Geometry check sheet. Reference: the model listing, model coordinates, mm. Give positions to 0.01 mm unless a question says otherwise; leave off trailing zeros. Write each loop counter-clockwise with the first axis right and the second up, starting at its lowest first coordinate (ties: lowest second). Pieces come first, ordered by that corner, then holes. Notation, with made-up numbers: (-39, 80.25) - (2, 80.25) arc R17 ccw to (2, 99.25) - close; hole circle Ø10 at (24.25, 77.5). An arc over 180 degrees is marked (long way). Use a Markdown table: item, result.
```python
from build123d import *

# Parameters (mm, degrees)
SKETCH1_W           = 82.55
SKETCH1_H           = 83.82
BOSS_EXTRUDE1_DEPTH = 19.05
SKETCH2_R           = 0.889
CUT_EXTRUDE1_DEPTH  = 71.083405489
FILLET1_R           = 2.54
SKETCH3_R           = 3.175
CUT_EXTRUDE2_DEPTH  = 38.1


with BuildPart() as part:
    # Sketch1 → Boss-Extrude1 (new, symmetric)
    with BuildSketch(Plane.XY):
        Rectangle(SKETCH1_W, SKETCH1_H)
    extrude(amount=BOSS_EXTRUDE1_DEPTH, both=True)

    # Sketch2 → Cut-Extrude1 (cut, through all)
    with BuildSketch(Plane.XY.offset(19.05)):
        with Locations((-28.575, 29.845)):
            Circle(SKETCH2_R)
        with Locations((28.575, 29.845)):
            Circle(SKETCH2_R)
        with Locations((28.575, 1.27)):
            Circle(SKETCH2_R)
        with Locations((-28.575, 1.27)):
            Circle(SKETCH2_R)
        with Locations((-19.685, 1.27)):
            Circle(SKETCH2_R)
        with Locations((19.685, 1.27)):
            Circle(SKETCH2_R)
    extrude(amount=-CUT_EXTRUDE1_DEPTH, mode=Mode.SUBTRACT)

    # Fillet1
    fillet1_edges = [part.edges().sort_by_distance(p)[0] for p in [
        (-41.275, 0, 19.05),
        (41.275, 0, 19.05),
        (-41.275, 0, -19.05),
        (41.275, 0, -19.05),
    ]]
    fillet(fillet1_edges, radius=FILLET1_R)

    # Sketch3 → Cut-Extrude2 (cut)
    with BuildSketch(Plane(origin=(0, 41.91, 0), x_dir=(1, 0, 0), z_dir=(0, 1, 0))):
        with Locations(Location((-6.35, 0, 0), (0, 0, 270))):
            Circle(SKETCH3_R)
        with Locations(Location((6.35, 0, 0), (0, 0, 270))):
            Circle(SKETCH3_R)
        with Locations(Location((19.05, 0, 0), (0, 0, 270))):
            Circle(SKETCH3_R)
        with Locations(Location((-19.05, 0, 0), (0, 0, 270))):
            Circle(SKETCH3_R)
    extrude(amount=-CUT_EXTRUDE2_DEPTH, mode=Mode.SUBTRACT)


solid = part.part
```
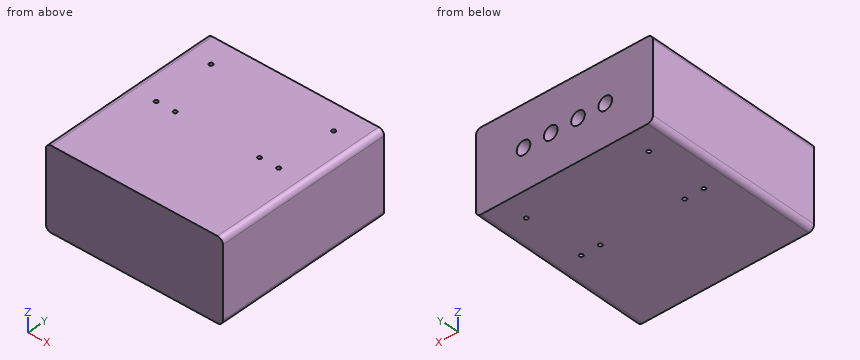
1) Section check C-C on x = -6.35. Record the boundary of the cut face in (y, z) (3 decimals).
Working result:
| item | result |
|---|---|
| outline | (-41.91, -19.05) - (41.91, -19.05) - (41.91, -3.175) - (3.81, -3.175) - (3.81, 3.175) - (41.91, 3.175) - (41.91, 19.05) - (-41.91, 19.05) - close |
2) Section check B-B on z = 0. Record the boundary of the cut face in (x, y) (3 decimals).
Working result:
| item | result |
|---|---|
| outline | (-41.275, -41.91) - (41.275, -41.91) - (41.275, 41.91) - (22.225, 41.91) - (22.225, 3.81) - (15.875, 3.81) - (15.875, 41.91) - (9.525, 41.91) - (9.525, 3.81) - (3.175, 3.81) - (3.175, 41.91) - (-3.175, 41.91) - (-3.175, 3.81) - (-9.525, 3.81) - (-9.525, 41.91) - (-15.875, 41.91) - (-15.875, 3.81) - (-22.225, 3.81) - (-22.225, 41.91) - (-41.275, 41.91) - close; hole circle Ø1.778 at (-28.575, 1.27); hole circle Ø1.778 at (-28.575, 29.845); hole circle Ø1.778 at (-19.685, 1.27); hole circle Ø1.778 at (19.685, 1.27); hole circle Ø1.778 at (28.575, 1.27); hole circle Ø1.778 at (28.575, 29.845) |
3) Section check A-A on y = 18. Record the boundary of the cut face in (x, z) (3 decimals).
Working result:
| item | result |
|---|---|
| outline | (-41.275, -16.51) arc R2.54 ccw to (-38.735, -19.05) - (38.735, -19.05) arc R2.54 ccw to (41.275, -16.51) - (41.275, 16.51) arc R2.54 ccw to (38.735, 19.05) - (-38.735, 19.05) arc R2.54 ccw to (-41.275, 16.51) - close; hole circle Ø6.35 at (-19.05, 0); hole circle Ø6.35 at (-6.35, 0); hole circle Ø6.35 at (6.35, 0); hole circle Ø6.35 at (19.05, 0) |
4) Depth check by flat-ended pin: P1, Ø3, axis at x = -5, z = 0.5, coming from the +Y side; P2, Ø1.1, axis at x = -19.685, y = 1.27, coming from the +Z side (3 decimals). Enter the tip coordinate at first touch or a pass-through.
Working result:
| item | result |
|---|---|
| P1 | stops at y = 3.81 |
| P2 | passes through |
5) Material ranges on L1, parallel to X at y = 14, z = 0 (3 decimals); L2, parallel to Y at x = -28, z = 15; L3, parallel to Z at x = 19, y = 17, recorded low to high. Write a range as from..to.
Working result:
| item | result |
|---|---|
| L1 | x = -41.275..-22.225, -15.875..-9.525, -3.175..3.175, 9.525..15.875, 22.225..41.275 |
| L2 | y = -41.91..0.59, 1.95..29.17, 30.52..41.91 |
| L3 | z = -19.05..-3.17, 3.17..19.05 |
